Input: part model. Units: mm. Frame: model coordinates. Coordinates: 2 decimals unless noted, no trailing zeros. Loops run counter-clockwise (first coordinate to the right, second up) from the corner with the lowest first, then second, coordinate; pieces in that order, holes last. Notation, with made-up numbers: M -10.75,64.25 L 46.25,64.25 A28 ccw 46.25,98.25 Z; hole C -4,27.25 d3. An arc over 180 degrees is marked long. Use a Markdown table: item, result. Add a question column.
1. Section A-A on y = -14. Output: boundary loops of the cut face in (x, z).
2. Draft query along Y for faces 1 (the flat face through (-63, 33, 3)), 2 (the cylindrical face through (15.46, 56.51, 1.48)), 3 (the cylindrical face through (-105.749, 79.982, 1.479)). Return one class per face: +Y half, -Y half, draft (parallel to the pull), parting line (faces both ways), or undercut.
3. Line query: L1, parallel to Y at x = -59.5, z = 2.55; L2, parallel to X at y = 90.5, z = 1.1; L3, parallel to Y at x = -120.5, z = 2. Output: solid intervals per line, ascending. Write a range as [from, to].
4. Section B-B on x = -16.5. Output: boundary loops of the cut face in (y, z).
5. Pin query (flat end, axial travel): pin 1 (13 mm diameter, centred on x = -109.43, y = 76.6, fed in from +Z); pin 2 (1 mm diameter, centred on y = 5, z = 0.5, fed in from -X); pin 3 (1 mm diameter, centred on y = 27, z = 1, fed in from +X). Return the tip coordinate at first contact, or that it passes through.
6. Section C-C on z = 1.1. Output: boundary loops of the cut face in (x, y).
```python
from build123d import *

# Parameters (mm, degrees)
F0_R     = 80.723069
F1_DEPTH = 3
F2_R     = 3
F3_DEPTH = 3
F5_D     = 10


with BuildPart() as f1:
    # F0 (on Top) → F1 (new body)
    with BuildSketch(Plane.XY):
        with Locations((-61.535046, 32.258771)):
            Circle(F0_R)
    extrude(amount=F1_DEPTH)

    # F2 (on face) → F3 (join)
    with BuildSketch(Plane.XY.offset(3)):
        with Locations((-128.833771, 47.312688)):
            Circle(F2_R)
    extrude(amount=-F3_DEPTH)

    # F5 (through all)
    with Locations(Plane.XY.offset(3)):
        with Locations((-109.434292, 76.603003)):
            Hole(F5_D / 2)


solid = f1.part
```
Answers below:
| question | item | result |
|---|---|---|
| 1 | outline | M -127.69,0 L 4.62,0 L 4.62,3 L -127.69,3 Z |
| 2 | face 1 | draft |
| 2 | face 2 | parting line |
| 2 | face 3 | undercut |
| 3 | L1 | y = [-48.44, 112.96] |
| 3 | L2 | x = [-117.43, -5.64] |
| 3 | L3 | y = [-22.87, 87.39] |
| 4 | outline | M -34.73,0 L 99.25,0 L 99.25,3 L -34.73,3 Z |
| 5 | pin 1 | stops at z = 3 |
| 5 | pin 2 | stops at x = -137.69 |
| 5 | pin 3 | stops at x = 19.05 |
| 6 | outline | C -61.54,32.26 d161.45; hole C -109.43,76.6 d10 |
